Geometry: final body of the model. Coordinates: model frame, mm. Give positions to 0.01 mm unless a question says otherwise; leave off trailing zeros. Write each loop counter-clockwise with the first axis right and the second up, starting at its lowest first coordinate (ties: lowest second). Pieces come first, ordered by that corner, then holes.
```python
from build123d import *

# Parameters (mm, degrees)
SKETCH1_W           = 50.8
SKETCH1_H           = 50.8
BOSS_EXTRUDE1_DEPTH = 50.8
SKETCH2_R           = 12.7
CUT_EXTRUDE1_DEPTH  = 50.8
SKETCH3_R           = 12.7
CUT_EXTRUDE2_DEPTH  = 50.8
SKETCH4_R           = 12.7
CUT_EXTRUDE3_DEPTH  = 50.8


with BuildPart() as part:
    # Sketch1 → Boss-Extrude1 (new body)
    with BuildSketch(Plane.XY):
        with Locations((25.4, 25.4)):
            Rectangle(SKETCH1_W, SKETCH1_H)
    extrude(amount=BOSS_EXTRUDE1_DEPTH)

    # Sketch2 → Cut-Extrude1 (cut)
    with BuildSketch(Plane.XY.offset(50.8)):
        with Locations((25.4, 25.4)):
            Circle(SKETCH2_R)
    extrude(amount=-CUT_EXTRUDE1_DEPTH, mode=Mode.SUBTRACT)

    # Sketch3 → Cut-Extrude2 (cut)
    with BuildSketch(Plane(origin=(0, 50.8, 0), x_dir=(1, 0, 0), z_dir=(0, 1, 0))):
        with Locations((25.4, -25.4)):
            Circle(SKETCH3_R)
    extrude(amount=-CUT_EXTRUDE2_DEPTH, mode=Mode.SUBTRACT)

    # Sketch4 → Cut-Extrude3 (cut)
    with BuildSketch(Plane.ZY):
        with Locations((25.4, 25.4)):
            Circle(SKETCH4_R)
    extrude(amount=-CUT_EXTRUDE3_DEPTH, mode=Mode.SUBTRACT)


solid = part.part
```
Item 1: Section A-A, the plane x = 25.4. Return the cut outline in (y, z), plus the area to 3 significant figures.
Found:
outline: (0, 0) - (12.7, 0) - (12.7, 12.7) - (0, 12.7) - close; (0, 38.1) - (12.7, 38.1) - (12.7, 50.8) - (0, 50.8) - close; (38.1, 0) - (50.8, 0) - (50.8, 12.7) - (38.1, 12.7) - close; (38.1, 38.1) - (50.8, 38.1) - (50.8, 50.8) - (38.1, 50.8) - close
area: 645 mm2
Item 2: Line query: L1, parallel to Z at x = 25, y = 4; L2, parallel to X at y = 10, z = 25.4. Output: solid intervals per line, ascending.
Found:
L1: z = 0 to 12.71, 38.09 to 50.8
L2: x = 0 to 12.7, 38.1 to 50.8
Item 3: Pull-direction query (Z, two-part tool) for faces 1 (the face through (44.3, 33.983, 16.04)), 2 (the face through (16.04, 6.5, 16.817)), 3 (the face through (14, 0, 19)), 4 (the face through (19, 37, 50.8)); classes: +Z half, -Z half, draft (parallel to the pull), parting line (faces both ways), or undercut.
Found:
face 1: undercut
face 2: undercut
face 3: draft
face 4: +Z half
Item 4: Section C-C, the plane y = 3.5. Return the cut outline in (x, z), plus the area to 3 significant figures.
Found:
outline: (0, 0) - (50.8, 0) - (50.8, 50.8) - (0, 50.8) - close; hole circle Ø25.4 at (25.4, 25.4)
area: 2,070 mm2
